from build123d import *

# Parameters (mm, degrees)
SKETCH1_W            = 15.8
SKETCH1_H            = 3.2
BOSS_EXTRUDE1_DEPTH  = 15.8
SKETCH2_R            = 2.4
BOSS_EXTRUDE2_DEPTH  = 1.6
LPATTERN1_COUNT      = 2
LPATTERN1_PITCH      = 8
LPATTERN1_COUNT_DIR2 = 4
LPATTERN1_PITCH_DIR2 = 8
SHELL1_T             = -1.2
SKETCH4_R            = 3.25
SKETCH4_R_2          = 2.4
BOSS_EXTRUDE3_DEPTH  = 1.8


with BuildPart() as part:
    # Sketch1 → Boss-Extrude1 (new body)
    with BuildSketch(Plane.XY):
        with Locations((7.9, 1.6)):
            Rectangle(SKETCH1_W, SKETCH1_H)
    extrude(amount=-BOSS_EXTRUDE1_DEPTH)

    # Sketch2 → Boss-Extrude2 (add)
    with BuildSketch(Plane(origin=(0, 3.2, 0), x_dir=(1, 0, 0), z_dir=(0, 1, 0))):
        with Locations(Location((3.9, 3.9, 0), (0, 0, 270))):
            Circle(SKETCH2_R)
    boss_extrude2 = extrude(amount=BOSS_EXTRUDE2_DEPTH)

    # LPattern1: Boss-Extrude2 2 × 4, 4 skipped
    with Locations(*[(j * LPATTERN1_PITCH_DIR2, 0, -i * LPATTERN1_PITCH) for i in range(LPATTERN1_COUNT) for j in range(LPATTERN1_COUNT_DIR2) if (i, j) not in ((0, 0), (0, 2), (0, 3), (1, 2), (1, 3))]):
        add(boss_extrude2)

    # Shell1
    shell1_openings = [part.faces().sort_by_distance(p)[0] for p in [
        (7.9, 0, -7.9),
    ]]
    offset(amount=SHELL1_T, openings=shell1_openings, kind=Kind.INTERSECTION)

    # Sketch4 → Boss-Extrude3 (add)
    with BuildSketch(Plane.XZ.offset(-2)):
        with Locations(Location((7.9, -7.9, 0), (0, 0, 90))):
            Circle(SKETCH4_R)
        with Locations(Location((7.9, -7.9, 0), (0, 0, 270))):
            Circle(SKETCH4_R_2, mode=Mode.SUBTRACT)
    extrude(amount=BOSS_EXTRUDE3_DEPTH)


solid = part.part
The listing builds one solid part. Answer for the finished solid, in the listing's coordinates (mm). A direction names the side the tool comes from. Give positions to 0.01 mm unless a question says otherwise; leave off trailing zeros. Write each loop counter-clockwise with the first axis right and the second up, starting at its lowest first coordinate (ties: lowest second). Pieces come first, ordered by that corner, then holes. Notation, with made-up numbers: (-34.5, -20.5) - (-6.5, -20.5) arc R16 cw to (-6.5, -3.5) - close; hole circle Ø4 at (25.5, 88). An arc over 180 degrees is marked (long way). One line per question, with ' | ' between items. Start each with the question number.
1. Determine the mould class of faces 1 (the face through (12, 3.6, -12)), 2 (the face through (0, 2, -8)), 3 (the face through (8, 2, -15.8)) for opening direction X: +X half, -X half, draft (parallel to the pull), parting line (faces both ways), or undercut.
2. Given P1, Ø2.5, axis at x = 3.5, z = -3.5, coming from the -Y side; P2, Ø7, axis at x = 6.5, z = -7.5, coming from the -Y side, each flat-ended and moving along its own axis, determine where each tip first touches the part or whether it passes through.
3. For faces 4 (the face through (8, 2, -8)), 5 (the face through (1.557, 3.989, -12.42)), 6 (the face through (1, 0, -8)), determine the directions among +Z, -Z, +X, -X, +Y, -Y from which every point of the face is accessible in a straight line to the end or side of a thin tool.
4. Section A-A, the plane y = 1.65 is taken. Determine the outline of the cut face in (x, z), then the cut area to 3 significant figures.
5. Section D-D, the plane z = -3.9 is taken. Determine the outline of the cut face in (x, y).
6. Section C-C, the plane x = 3.9 is taken. Determine the outline of the cut face in (y, z), then the cut area to 3 significant figures.
7. Section B-B, the plane y = 2.65 is taken. Determine the outline of the cut face in (x, z).
8. Straight lines are drawn through the part: line 1 (X direction, y = 3.15, z = -11.9); line 2 (Z direction, x = 3.9, y = 2.75); line 3 (Z direction, x = 8.5, y = 0.9). For each, find the intervals that lie inside material, in ascending order.
Result:
1) face 1: undercut | face 2: -X half | face 3: draft
2) P1: stops at y = 2 | P2: stops at y = 0.2
3) face 4: -Y | face 5: +Y | face 6: +Z, -Z, +X, -X, -Y
4) outline: (0, -15.8) - (15.8, -15.8) - (15.8, 0) - (0, 0) - close; circle Ø6.5 at (7.9, -7.9); hole (1.2, -14.6) - (14.6, -14.6) - (14.6, -1.2) - (1.2, -1.2) - close; hole circle Ø4.8 at (7.9, -7.9) | area: 85.2 mm2
5) outline: (0, 0) - (1.2, 0) - (1.2, 2) - (2.7, 2) - (2.7, 3.6) - (5.1, 3.6) - (5.1, 2) - (10.7, 2) - (10.7, 3.6) - (13.1, 3.6) - (13.1, 2) - (14.6, 2) - (14.6, 0) - (15.8, 0) - (15.8, 3.2) - (14.3, 3.2) - (14.3, 4.8) - (9.5, 4.8) - (9.5, 3.2) - (6.3, 3.2) - (6.3, 4.8) - (1.5, 4.8) - (1.5, 3.2) - (0, 3.2) - close
6) outline: (0, -15.8) - (3.2, -15.8) - (3.2, -14.3) - (4.8, -14.3) - (4.8, -9.5) - (3.2, -9.5) - (3.2, -6.3) - (4.8, -6.3) - (4.8, -1.5) - (3.2, -1.5) - (3.2, 0) - (0, 0) - (0, -1.2) - (2, -1.2) - (2, -2.7) - (3.6, -2.7) - (3.6, -5.1) - (2, -5.1) - (2, -10.7) - (3.6, -10.7) - (3.6, -13.1) - (2, -13.1) - (2, -14.6) - (0, -14.6) - close | area: 31.4 mm2
7) outline: (0, -15.8) - (15.8, -15.8) - (15.8, 0) - (0, 0) - close; hole circle Ø2.4 at (3.9, -11.9); hole circle Ø2.4 at (3.9, -3.9); hole circle Ø2.4 at (11.9, -11.9); hole circle Ø2.4 at (11.9, -3.9)
8) line 1: x = 0 to 2.7, 5.1 to 10.7, 13.1 to 15.8 | line 2: z = -15.8 to -13.1, -10.7 to -5.1, -2.7 to 0 | line 3: z = -15.8 to -14.6, -11.09 to -10.22, -5.58 to -4.71, -1.2 to 0
